Autodesk Inventor part; units mm, degrees
ref_plane "YZ Plane" through (0, 0, 0) normal (1, 0, 0) x (0, 1, 0)
ref_plane "XZ Plane" through (0, 0, 0) normal (0, 1, 0) x (-1, 0, 0)
ref_plane "XY Plane" through (0, 0, 0) normal (0, 0, 1) x (1, 0, 0)
sketch "Sketch1" plane through (0, 0, 0) normal (0, 1, 0) x (-1, 0, 0)
  line L0 (-12, -24.5) -> (12, -24.5)
  line L1 (12, -24.5) -> (12, 24.5)
  line L2 (12, 24.5) -> (-12, 24.5)
  line L3 (-12, 24.5) -> (-12, -24.5)
  line L4 (-12, -24.5) -> (12, 24.5) construction
  line L5 (12, -24.5) -> (-12, 24.5) construction
  point P0 (0, 0)
  dimension "d0" = 24
  dimension "d1" = 49
extrude "Extrusion1" add sketch "Sketch1" along normal blind 5.4 and the other way blind 13.8
shell "Shell1" thickness 1.5 removed faces 1 at (4, 5.4, 8.1667)
sketch "Sketch2" plane through (-12, -13.8, 24.5) normal (-1, 0, 0) x (0, 0, 1)
  line L0 (0, 0) -> (0, 19.2)
  line L1 (-49, 19.2) -> (-49, 0)
  line L2 (0, 0) -> (-49, 0)
  line L3 (-49, 0) -> (-49, 19.2)
  line L4 (-49, 1.5) -> (0, 1.5)
  circle A0 centre (-29.15, 5) radius 3.5
  line L5 (-24.5, 13.8) -> (-24.5, 1.5)
  line L6 (-24.5, 11) -> (0, 11)
  line L7 (-24.5, 13) -> (-49, 13)
  circle A1 centre (-19.85, 5) radius 3.5
  point P0 (-24.5, 13.8)
  dimension "d7" = 1.5
  dimension "d8" = 3.5
  dimension "d9" = 7
  dimension "d10" = 4.65
  dimension "d11" = 7
  dimension "d12" = 1.15
extrude "Extrusion2" cut sketch "Sketch2" against normal blind 5.4 contours A1 | A0
sketch "Sketch3" plane through (0, 5.4, 0) normal (0, 1, 0) x (1, 0, 0)
  line L0 (-10.5, 23) -> (10.5, 23)
  line L1 (10.5, 23) -> (10.5, -23)
  line L2 (10.5, -23) -> (-10.5, -23)
  line L3 (-12, 24.5) -> (-12, -24.5)
  line L4 (-12, -24.5) -> (12, -24.5)
  line L5 (12, -24.5) -> (12, 24.5)
  line L6 (12, 24.5) -> (-12, 24.5)
  line L7 (12, 24.5) -> (-12, 24.5)
  line L8 (-12, 24.5) -> (-12, -24.5)
  line L9 (-12, -24.5) -> (12, -24.5)
  line L10 (12, -24.5) -> (12, 24.5)
  circle A0 centre (0, 12.5) radius 8.5
  circle A1 centre (0, -12.5) radius 8.5
  point P0 (0, 0)
  dimension "d15" = 17
  dimension "d16" = 2
  dimension "d17" = 2
  dimension "d18" = 17
  dimension "d19" = 2
  dimension "d20" = 2
extrude "Extrusion3" add sketch "Sketch3" along normal blind 1.5
properties part number "carcasaXeotype_ULTRASONIC"
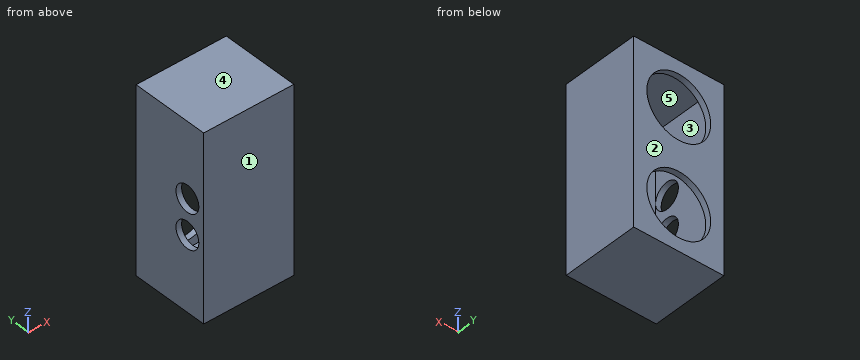
The listing builds one solid part. Answer for the finished solid, in the listing's coordinates (mm). Face numbers are marked on the shaded views. A direction names the side the tool comes from. Round coordinates to 2 decimals unless told otherwise and drop trailing zeros. Loops run counter-clockwise (first coordinate to the right, second up) from the corner with the lowest first, then second, coordinate; pieces in that order, holes last.
Q1. Section B-B, the plane x = 0 is taken. Determine the outline of the cut face in (y, z).
Q2. For a pull along Y with two mould halves and no side action, classify the marked faces 1, 2 and 3 as released by +Y, released by -Y, zero draft, split by the parting line, or undercut.
Q3. Section D-D, the plane x = 9.5 is taken. Determine the outline of the cut face in (y, z), then the cut area to 3 significant figures.
Q4. Section C-C, the plane y = -10.75 is taken. Determine the outline of the cut face in (x, z).
Q5. Given pin 1 Ø3 at (x, z) = (4.5, -10) entering from +Y; pin 2 Ø4 at (y, z) = (-8.8, 4.65) entering from -X, each flat-ended and moving along its own axis, determine where each tip first touches the part or whether it passes through.
Q6. Which of the six approach directions +Z, -Z, +X, -X, +Y, -Y give full straight-line access (tool end or side, diameter ignored) to the marked faces 4 and 5?
Q7. Find the intervals of material crossed by line 1 (Z direction, x = 0, y = 6.2); line 2 (Z direction, x = -11.6, y = -8.8); line 3 (X direction, y = -7.5, z = 11), in increasing order.
Q8. Section A-A, the plane y = -0.25 is taken. Determine the outline of the cut face in (x, z).
Completed:
1. outline: (-13.8, -24.5) - (6.9, -24.5) - (6.9, -21) - (5.4, -21) - (5.4, -23) - (-12.3, -23) - (-12.3, 23) - (5.4, 23) - (5.4, 21) - (6.9, 21) - (6.9, 24.5) - (-13.8, 24.5) - close; (5.4, -4) - (6.9, -4) - (6.9, 4) - (5.4, 4) - close
2. face 1: released by -Y
2. face 2: released by +Y
2. face 3: undercut
3. outline: (-13.8, -24.5) - (6.9, -24.5) - (6.9, 24.5) - (-13.8, 24.5) - close; hole (-12.3, -23) - (5.4, -23) - (5.4, 23) - (-12.3, 23) - close
3. area: 200 mm2
4. outline: (-12, -24.5) - (12, -24.5) - (12, 24.5) - (-12, 24.5) - (-12, 7.56) - (-10.5, 7.56) - (-10.5, 23) - (10.5, 23) - (10.5, -23) - (-10.5, -23) - (-10.5, -7.56) - (-12, -7.56) - close; (-12, -1.74) - (-10.5, -1.74) - (-10.5, 1.74) - (-12, 1.74) - close
5. pin 1: stops at y = -12.3
5. pin 2: stops at x = 10.5
6. face 4: +Z, +X, -X, +Y, -Y
6. face 5: none
7. line 1: z = -24.5 to -21, -4 to 4, 21 to 24.5
7. line 2: z = -24.5 to -8.15, -1.15 to 1.15, 8.15 to 24.5
7. line 3: x = -12 to -10.5, 10.5 to 12
8. outline: (-12, -24.5) - (12, -24.5) - (12, 24.5) - (-12, 24.5) - close; hole (-10.5, -23) - (10.5, -23) - (10.5, 23) - (-10.5, 23) - close
